Geometry: see drawing. Coordinates: mm, zero at the bounding-box minimum. Coordinates: 2 decimals unless noted, no trailing zeros. Order: outer loops, then holes, each group sorted by start corner. A loop starts at its lowest first (then second) coordinate and runs counter-clockwise, first axis right, second up. Notation, with made-up numbers: (-33, -26.75) -> (-3, -26.75) arc R21 cw to (-3, 3.25) -> close; hole circle Ø9 at (29, 73). An arc over 180 degrees is marked (long way). Write each question's results on one line, items separated by ' | '. Start each with the question number.
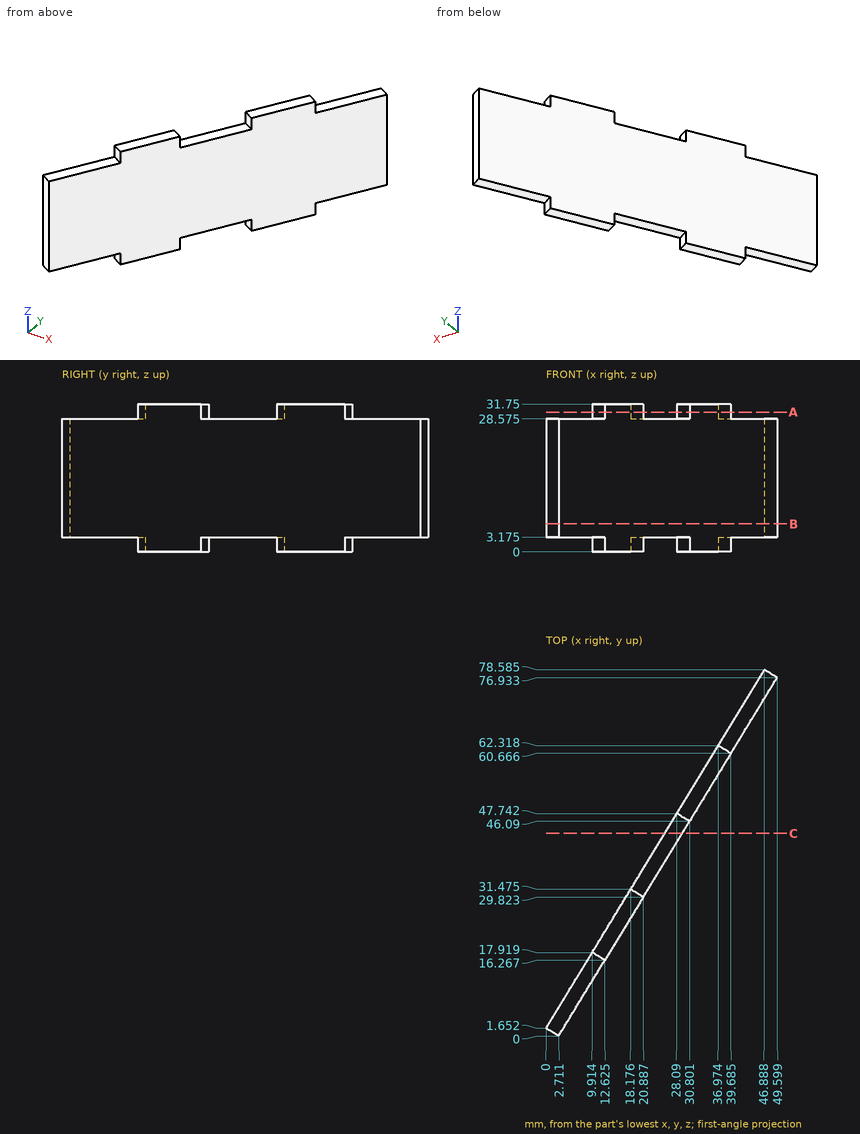
(1) Section A-A on z = 30. Return the cut outline in (x, y) (1 decimal).
(2) Section C-C on y = 43.5. Return the cut outline in (x, z) (1 decimal).
(3) Line query: L1, parallel to X at y = 69, z = 19 (1 decimal); L2, parallel to Y at x = 46, z = 28 (1 decimal); L3, parallel to X at y = 45.5, z = 17.5 (1 decimal). Output: solid intervals per line, ascending.
(4) First-contact query: P1, Ø14, axis at x = 42, y = 72.5, coming from the -Z side (3 decimals); P2, Ø6, axis at x = 22, z = 16.5, coming from the +Y side; P3, Ø5, axis at x = 20.5, z = 10, coming from the +Y side. Flat tips, straight axial feed; report the tip coordinate or a pass-through.
(5) Section B-B on z = 6. Return the cut outline in (x, y) (1 decimal), then the cut area to 3 significant figures.
Results list:
1) outline: (9.9, 17.9) -> (12.6, 16.3) -> (20.9, 29.8) -> (18.2, 31.5) -> close; (28.1, 47.7) -> (30.8, 46.1) -> (39.7, 60.7) -> (37, 62.3) -> close
2) outline: (25.5, 3.2) -> (29.2, 3.2) -> (29.2, 28.6) -> (25.5, 28.6) -> close
3) L1: x = 41 to 44.8 | L2: y = 71 to 77.1 | L3: x = 26.7 to 30.4
4) P1: stops at z = 3.175 | P2: stops at y = 42.67 | P3: stops at y = 39.39
5) outline: (0, 1.7) -> (2.7, 0) -> (49.6, 76.9) -> (46.9, 78.6) -> close | area: 286 mm²
